Can you work these out from the model? Positions are in its coordinate system, mm. Face numbers are marked on the shaded views. A direction names the side the tool comes from. Give positions to 0.01 mm unless a question says otherwise; leave off trailing zeros. Loops run counter-clockwise (first coordinate to the right, second up) from the corner with the lowest first, then second, coordinate; pieces in that order, holes last. Notation, with made-up numbers: M 38.25,-11 L 89.25,-11 A21 ccw 89.25,-5 Z; hole C 45,17 d8. An arc over 180 degrees is marked long. Use CSV: the item, a comma, the result in double quotes.
from build123d import *

# Parameters (mm, degrees)
F0_R     = 7
F0_R_2   = 2.5
F1_DEPTH = 5
F2_R     = 5
F2_R_2   = 2.5
F3_DEPTH = 0.5
F4_R     = 5
F4_R_2   = 2.5
F5_DEPTH = 0.5


with BuildPart() as f1:
    # F0 (on Front) → F1 (new body)
    with BuildSketch(Plane.XZ):
        Circle(F0_R)
        Circle(F0_R_2, mode=Mode.SUBTRACT)
    extrude(amount=F1_DEPTH)

    # F2 (on face) → F3 (join)
    with BuildSketch(Plane.XZ.offset(5)):
        Circle(F2_R)
        Circle(F2_R_2, mode=Mode.SUBTRACT)
    extrude(amount=F3_DEPTH)

    # F4 (on face) → F5 (join)
    with BuildSketch(Plane(origin=(0, 0, 0), x_dir=(-1, 0, 0), z_dir=(0, 1, 0))):
        Circle(F4_R)
        Circle(F4_R_2, mode=Mode.SUBTRACT)
    extrude(amount=F5_DEPTH)


solid = f1.part
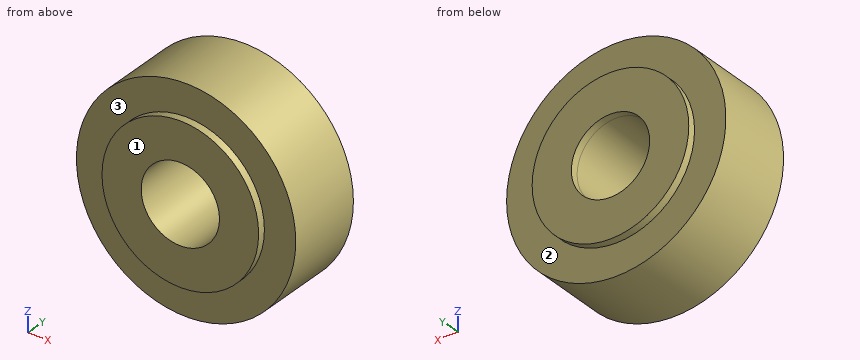
Q1. For the marked faces 1, 2 and 3, which set-ups out of +Z, -Z, +X, -X, +Y, -Y let a thin tool reach every point of the face, with its end or its side?
Model answer:
face 1,"+Z, -Z, +X, -X, -Y"
face 2,"+Y"
face 3,"-Y"
Q2. I want a section at D-D, the plane x = -3.25. Please give me the cut outline in (y, z), then the cut area to 3 significant figures.
Model answer:
outline,"M -5.5,-3.8 L -5,-3.8 L -5,-6.2 L 0,-6.2 L 0,-3.8 L 0.5,-3.8 L 0.5,3.8 L 0,3.8 L 0,6.2 L -5,6.2 L -5,3.8 L -5.5,3.8 Z"
area,"69.6 mm2"
Q3. I'm going to push flat-ended pins straight in: P1, Ø1.5, axis at x = 1.5, y = -4, coming from the -Z side; P2, Ø8, axis at x = 1.5, z = 0, coming from the -Y side. Where does each tip first touch, or does it pass through?
Model answer:
P1,"z = -6.96"
P2,"y = -5.5"
Q4. I want a section at C-C, the plane y = -4.1. Please give me the cut outline in (x, z), then the cut area to 3 significant figures.
Model answer:
outline,"C 0,0 d14; hole C 0,0 d5"
area,"134 mm2"
Q5. Please list where these lines run through material, in increasing order: L1, parallel to Z at x = 0, y = -4; L2, parallel to Z at x = 0, y = 0.3; L3, parallel to Y at x = -4.5, z = -3.5. Write a range as from..to.
Model answer:
L1,"-7..-2.5, 2.5..7"
L2,"-5..-2.5, 2.5..5"
L3,"-5..0"
Q6. I want a section at A-A, the plane x = 0. Please give me the cut outline in (y, z), then the cut area to 3 significant figures.
Model answer:
outline,"M -5.5,-5 L -5,-5 L -5,-7 L 0,-7 L 0,-5 L 0.5,-5 L 0.5,-2.5 L -5.5,-2.5 Z; M -5.5,2.5 L 0.5,2.5 L 0.5,5 L 0,5 L 0,7 L -5,7 L -5,5 L -5.5,5 Z"
area,"50.0 mm2"
Q7. I want a section at B-B, the plane z = 0. Please give me the cut outline in (x, y).
Model answer:
outline,"M -7,-5 L -5,-5 L -5,-5.5 L -2.5,-5.5 L -2.5,0.5 L -5,0.5 L -5,0 L -7,0 Z; M 2.5,-5.5 L 5,-5.5 L 5,-5 L 7,-5 L 7,0 L 5,0 L 5,0.5 L 2.5,0.5 Z"
